Geometry check sheet. Reference: drawing and pictorial views, mm from the part's lowest x, y, z. Give positions to 0.01 mm unless a question says otherwise; leave off trailing zeros. Order: outer loops, then holes, each group sorted by start corner. A loop starts at its lowest first (then second) coordinate and runs counter-clockwise, first axis right, second up. Notation, with made-up numbers: (37.25, -27.75) -> (96.25, -27.75) arc R25 cw to (96.25, -0.75) -> close; hole circle Ø7 at (-19.5, 64.25). An arc over 180 degrees is marked (long way). Write each question's results on one line, items separated by ' | '. Start each with the question number.
1. Depth check by flat-ended pin: pin 1 Ø1.5 at (x, y) = (39, 1.5) entering from -Z; pin 2 Ø1.5 at (y, z) = (1.5, 36) entering from -X. Enter the tip coordinate at first touch or a pass-through.
2. Material ranges on L1, parallel to X at y = 0.85, z = 66.5; L2, parallel to Z at x = 91, y = 1.25; L3, parallel to X at y = 2.3, z = 55.5, recorded low to high. Write a range as from..to.
3. Cross-section at D-D, the plane x = 18. Enter the section's corners in (y, z).
4. Cross-section at C-C, the plane y = 1.4. Enter the section's corners in (x, z).
5. Cross-section at B-B, the plane z = 48.5. Enter the section's corners in (x, y), then the cut area to 3 significant figures.
6. Cross-section at A-A, the plane x = 4. Enter the section's corners in (y, z).
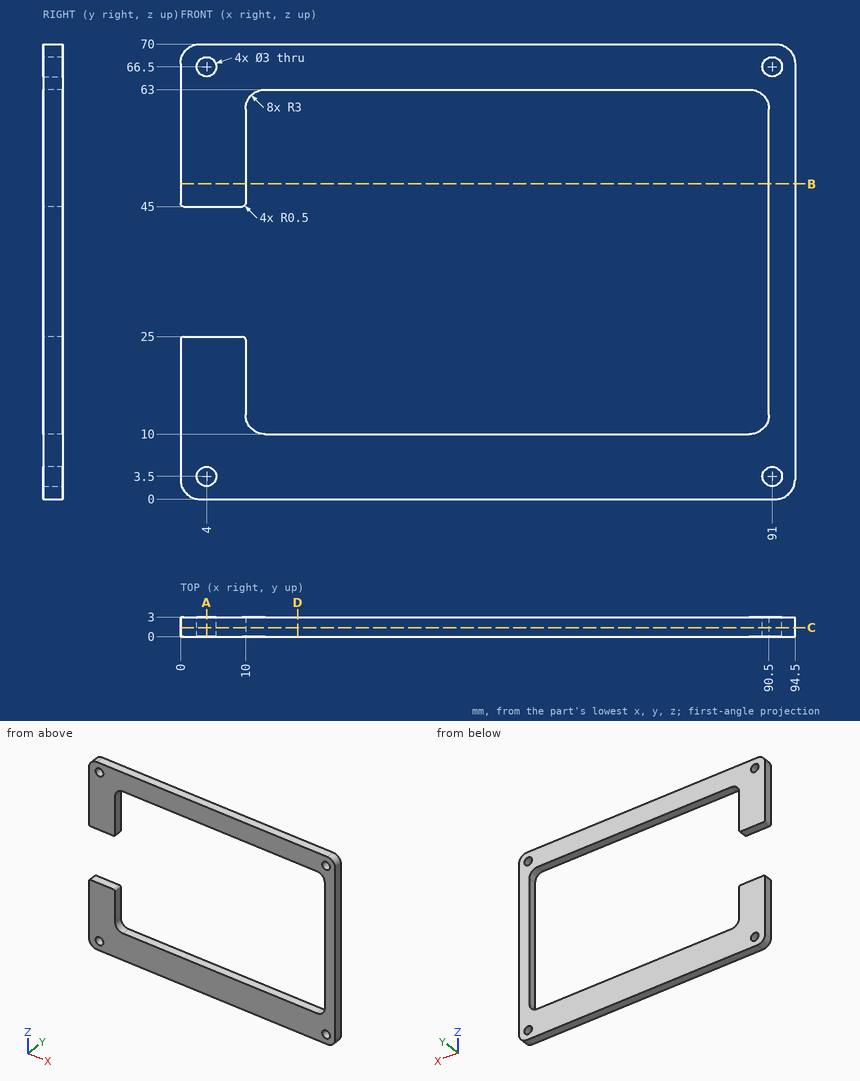
Results below:
1) pin 1: stops at z = 0 | pin 2: stops at x = 90.5
2) L1: x = 0..2.5, 5.5..89.5, 92.5..94.5 | L2: z = 0..2, 5..65, 68..70 | L3: x = 0..10, 90.5..94.5
3) outline: (0, 0) -> (3, 0) -> (3, 10) -> (0, 10) -> close; (0, 63) -> (3, 63) -> (3, 70) -> (0, 70) -> close
4) outline: (0, 3) arc R3 ccw to (3, 0) -> (91.5, 0) arc R3 ccw to (94.5, 3) -> (94.5, 67) arc R3 ccw to (91.5, 70) -> (3, 70) arc R3 ccw to (0, 67) -> (0, 45.5) arc R0.5 ccw to (0.5, 45) -> (9.5, 45) arc R0.5 ccw to (10, 45.5) -> (10, 60) arc R3 cw to (13, 63) -> (87.5, 63) arc R3 cw to (90.5, 60) -> (90.5, 13) arc R3 cw to (87.5, 10) -> (13, 10) arc R3 cw to (10, 13) -> (10, 24.5) arc R0.5 ccw to (9.5, 25) -> (0.5, 25) arc R0.5 ccw to (0, 24.5) -> close; hole circle Ø3 at (4, 3.5); hole circle Ø3 at (4, 66.5); hole circle Ø3 at (91, 3.5); hole circle Ø3 at (91, 66.5)
5) outline: (0, 0) -> (10, 0) -> (10, 3) -> (0, 3) -> close; (90.5, 0) -> (94.5, 0) -> (94.5, 3) -> (90.5, 3) -> close | area: 42.0 mm²
6) outline: (0, 0) -> (3, 0) -> (3, 2) -> (0, 2) -> close; (0, 5) -> (3, 5) -> (3, 25) -> (0, 25) -> close; (0, 45) -> (3, 45) -> (3, 65) -> (0, 65) -> close; (0, 68) -> (3, 68) -> (3, 70) -> (0, 70) -> close
